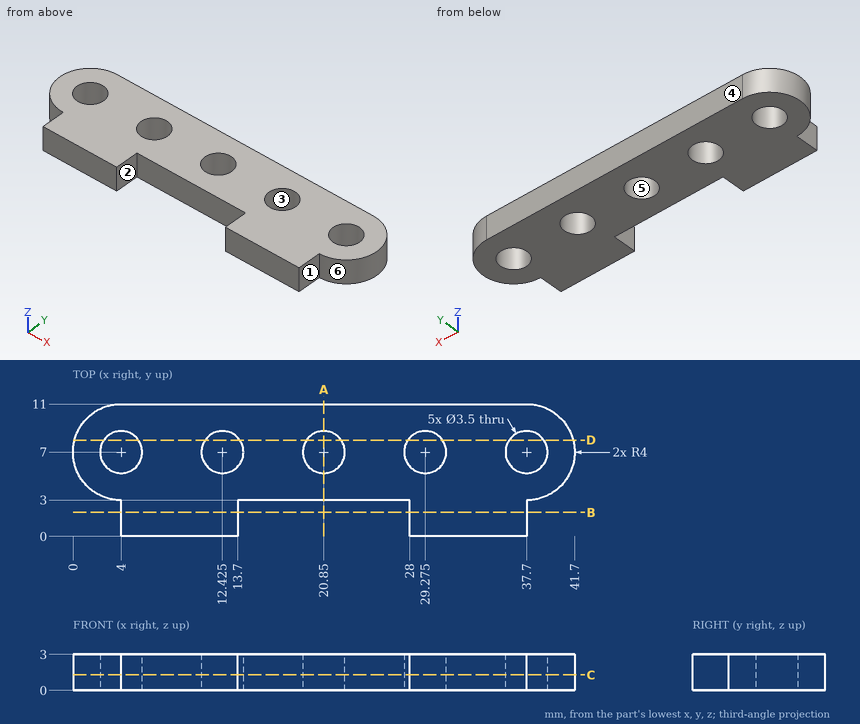
Could you check a few things on this drawing? It's one solid part, dimensions in mm from its lowest x, y, z. A direction names the side the tool comes from. Coordinates: 2 decimals unless noted, no trailing zeros. Order: outer loops, then holes, each group sorted by start corner. A loop starts at its lowest first (then second) coordinate and runs counter-clockwise, first axis right, second up. Notation, with made-up numbers: M 2,26.25 L 37,26.25 A34 cw 37,57.25 Z; hole C 38,60 d2. An arc over 180 degrees is marked long. Use a Markdown table: item, result. Add a question column.
Q1. I want a section at B-B on y = 2. List the corners of the cut face in (x, z) for me.
Q2. I want a section at C-C on z = 1.3. List the corners of the cut face in (x, y) for me (3 decimals), then the cut area to 3 significant figures.
Q3. I want a section at D-D on y = 8. List the corners of the cut face in (x, z) for me.
Q4. We'd pull the mould along Y, two halves only. Please class the marked faces 4, 5 and 6: pulls with the +Y half, pulls with the -Y half, needs draft (parallel to the pull), parting line crosses it, or undercut.
Q5. I want a section at A-A on x = 20.85. List the corners of the cut face in (y, z) for me.
Q6. Which directions (+Z, -Z, +X, -X, +Y, -Y) give clear straight access to the entire face, cutting with the end or side of a thin tool? Please do the marked faces 1, 2 and 3.
Q7. If I drill on L1, parallel to X at y = 8.5, z = 2.35; L2, parallel to X at y = 2, z = 0.55; L3, parallel to X at y = 6.25, z = 1.55, over which ranges is the centre line in solid material (lowest first)?
Q8. I'm going to push flat-ended pins straight in: pin 1 (0.9 mm diameter, centred on y = 1, z = 1.5, fed in from -X); pin 2 (3 mm diameter, centred on x = 29.275, y = 7, fed in from -Z); pin 3 (0.9 mm diameter, centred on x = 18.5, z = 2, fed in from -Y); pin 4 (2 mm diameter, centred on x = 11, y = 8.5, fed in from -Z). Where does each tip first touch, or does it pass through?
Checked values:
| question | item | result |
|---|---|---|
| 1 | outline | M 4,0 L 13.7,0 L 13.7,3 L 4,3 Z; M 28,0 L 37.7,0 L 37.7,3 L 28,3 Z |
| 2 | outline | M 4,0 L 13.7,0 L 13.7,3 L 28,3 L 28,0 L 37.7,0 L 37.7,3 A4 ccw 37.7,11 L 4,11 A4 ccw 4,3 Z; hole C 4,7 d3.5; hole C 12.425,7 d3.5; hole C 20.85,7 d3.5; hole C 29.275,7 d3.5; hole C 37.7,7 d3.5 |
| 2 | area | 330 mm² |
| 3 | outline | M 0.13,0 L 2.56,0 L 2.56,3 L 0.13,3 Z; M 5.44,0 L 10.99,0 L 10.99,3 L 5.44,3 Z; M 13.86,0 L 19.41,0 L 19.41,3 L 13.86,3 Z; M 22.29,0 L 27.84,0 L 27.84,3 L 22.29,3 Z; M 30.71,0 L 36.26,0 L 36.26,3 L 30.71,3 Z; M 39.14,0 L 41.57,0 L 41.57,3 L 39.14,3 Z |
| 4 | face 4 | pulls with the +Y half |
| 4 | face 5 | undercut |
| 4 | face 6 | parting line crosses it |
| 5 | outline | M 3,0 L 5.25,0 L 5.25,3 L 3,3 Z; M 8.75,0 L 11,0 L 11,3 L 8.75,3 Z |
| 6 | face 1 | +Z, -Z, +X, -Y |
| 6 | face 2 | +Z, -Z, -Y |
| 6 | face 3 | +Z, -Z |
| 7 | L1 | 0.29 to 3.1, 4.9 to 11.52, 13.33 to 19.95, 21.75 to 28.37, 30.18 to 36.8, 38.6 to 41.41 |
| 7 | L2 | 4 to 13.7, 28 to 37.7 |
| 7 | L3 | 0.07 to 2.42, 5.58 to 10.84, 14.01 to 19.27, 22.43 to 27.69, 30.86 to 36.12, 39.28 to 41.63 |
| 8 | pin 1 | x = 4 |
| 8 | pin 2 | through |
| 8 | pin 3 | y = 3 |
| 8 | pin 4 | z = 0 |
